Build history of the part. All positions in model axes, mm. A direction names the side the tool comes from. Coordinates: 2 decimals unless noted, no trailing zeros. Loops run counter-clockwise (first coordinate to the right, second up) from the corner with the lowest first, then second, coordinate; pieces in that order, holes last.
Item 1: 3-axis set-ups, long thin cutter, end or side, ignore diameter. For faces 1 (the face through (137, 40, -62)), 2 (the face through (-5, 65, 53)), 3 (the face through (19, 30, 1)), 4 (the face through (107, 40, 60)): which of +Z, -Z, +X, -X, +Y, -Y reach the whole face in a straight line?
Item 2: Cut at A-A (y = 47.5). List the corners of the cut face in (x, z), and give its area (3 significant figures).
Item 3: Cut at D-D (y = 17.5). List the corners of the cut face in (x, z), and give its area (3 significant figures).
Item 4: Cut at B-B (x = 45). List the corners of the cut face in (y, z), and give its area (3 significant figures).
Item 5: Drill centre lines: line 1 along X through (y, z) = (9, 13.5); line 2 along Y through (x, z) = (172, 9); line 3 along X through (y, z) = (-32.5, 14.5). Where is each one in solid material? Low to high.
Item 6: Cut at C-C (z = 33). List the corners of the cut face in (x, y), and give its area (3 significant figures).
Item 7: Mould opens along Y. For faces 5 (the face through (118, 35, 1)), 6 (the face through (167.5, 42.7, 62)), 7 (the face through (0, 15, 1)) say: released by +Y, released by -Y, zero draft, split by the parting line, or undercut.
Item 8: Flat gauge pins, fed straight in: pin 1 (1.5 mm diameter, centred on x = 83, z = 20.5, fed in from +Y); pin 2 (1.8 mm diameter, centred on x = 93.5, y = 41, fed in from -Z); pin 3 (5.5 mm diameter, centred on x = 183, y = 40, fed in from -Z); pin 4 (2.5 mm diameter, centred on x = 107.5, z = -63.5, fed in from -Y). Where does each tip first touch, or does it go through?
from build123d import *

# Parameters (mm, degrees)
EXTRUDE_1_DEPTH        = 65
SKETCH_5_W             = 5
SKETCH_5_H             = 5
CUT_EXTRUDE_1_DEPTH    = 3
SKETCH_7_W             = 5
SKETCH_7_H             = 23
EXTRUDE_2_DEPTH        = 40
FILLET_1_R             = 1
SKETCH_8_W             = 6
SKETCH_8_H             = 6
CUT_EXTRUDE_2_DEPTH    = 2
FILLET_1_OF_MIRROR_3_R = 1


with BuildPart() as part:
    # 草图1 → 凸台-拉伸1 (new body)
    with BuildSketch(Plane.XY):
        Polygon((190, 35), (190, 45), (-10, 45), (-10, 0), (0, 0), (0, 30), (39, 30), (39, -45), (49, -45), (49, 35), align=None)
    extrude_1 = extrude(amount=EXTRUDE_1_DEPTH)

    # 草图5 → 切除-拉伸1 (cut)
    with BuildSketch(Plane.XY.offset(65)):
        with Locations((167.5, 40)):
            Rectangle(SKETCH_5_W, SKETCH_5_H)
        with Locations((182.5, 40)):
            Rectangle(SKETCH_5_W, SKETCH_5_H)
        with Locations((152.5, 40)):
            Rectangle(SKETCH_5_W, SKETCH_5_H)
        with Locations((137.5, 40)):
            Rectangle(SKETCH_5_W, SKETCH_5_H)
        with Locations((122.5, 40)):
            Rectangle(SKETCH_5_W, SKETCH_5_H)
        with Locations((107.5, 40)):
            Rectangle(SKETCH_5_W, SKETCH_5_H)
        with Locations((92.5, 40)):
            Rectangle(SKETCH_5_W, SKETCH_5_H)
    cut_extrude_1 = extrude(amount=-CUT_EXTRUDE_1_DEPTH, mode=Mode.SUBTRACT)

    # 草图7 → 凸台-拉伸2 (add)
    with BuildSketch(Plane(origin=(0, 45, 0), x_dir=(1, 0, 0), z_dir=(0, 1, 0))):
        with Locations((-7.5, -53.5)):
            Rectangle(SKETCH_7_W, SKETCH_7_H)
    extrude_2 = extrude(amount=EXTRUDE_2_DEPTH)

    # 圆角1
    fillet_1_edges = [part.edges().sort_by_distance(p)[0] for p in [
        (-5, 65, 65),
        (-7.5, 85, 65),
        (-5, 0, 65),
        (0, 15, 65),
        (190, 45, 32.5),
        (190, 35, 32.5),
        (19.5, 30, 65),
        (39, -7.5, 65),
        (44, -45, 65),
        (49, -5, 65),
        (119.5, 35, 65),
        (190, 40, 65),
        (92.5, 45, 65),
        (-10, 42.5, 65),
    ]]
    fillet(fillet_1_edges, radius=FILLET_1_R)

    # 草图8 → 切除-拉伸2 (cut)
    with BuildSketch(Plane.XY.offset(62)):
        with Locations((182.5, 40)):
            Rectangle(SKETCH_8_W, SKETCH_8_H)
        with Locations((167.5, 40)):
            Rectangle(SKETCH_8_W, SKETCH_8_H)
        with Locations((152.5, 40)):
            Rectangle(SKETCH_8_W, SKETCH_8_H)
        with Locations((137.5, 40)):
            Rectangle(SKETCH_8_W, SKETCH_8_H)
        with Locations((122.5, 40)):
            Rectangle(SKETCH_8_W, SKETCH_8_H)
        with Locations((107.5, 40)):
            Rectangle(SKETCH_8_W, SKETCH_8_H)
        with Locations((92.5, 40)):
            Rectangle(SKETCH_8_W, SKETCH_8_H)
    extrude(amount=-CUT_EXTRUDE_2_DEPTH, mode=Mode.SUBTRACT)

    # 镜向3: 凸台-拉伸1, 切除-拉伸1, 凸台-拉伸2 across plane
    add(extrude_1.mirror(Plane.XY))
    add(cut_extrude_1.mirror(Plane.XY), mode=Mode.SUBTRACT)
    add(extrude_2.mirror(Plane.XY))

    # 圆角1 of 镜向3
    fillet_1_of_mirror_3_edges = [part.edges().sort_by_distance(p)[0] for p in [
        (-5, 65, -65),
        (-7.5, 85, -65),
        (-5, 0, -65),
        (0, 15, -65),
        (190, 45, -32.5),
        (190, 35, -32.5),
        (19.5, 30, -65),
        (39, -7.5, -65),
        (44, -45, -65),
        (49, -5, -65),
        (119.5, 35, -65),
        (190, 40, -65),
        (92.5, 45, -65),
        (-10, 42.5, -65),
    ]]
    fillet(fillet_1_of_mirror_3_edges, radius=FILLET_1_OF_MIRROR_3_R)


solid = part.part
Filled sheet:
1. face 1: -Z
1. face 2: +Z, -Z, +X, +Y
1. face 3: +Z, -Z, -Y
1. face 4: none
2. outline: (-10, -64) arc R1 ccw to (-9, -65) - (-6, -65) arc R1 ccw to (-5, -64) - (-5, -42) - (-10, -42) - close; (-10, 42) - (-5, 42) - (-5, 64) arc R1 ccw to (-6, 65) - (-9, 65) arc R1 ccw to (-10, 64) - close
2. area: 229 mm2
3. outline: (-10, -64) arc R1 ccw to (-9, -65) - (-1, -65) arc R1 ccw to (0, -64) - (0, 64) arc R1 ccw to (-1, 65) - (-9, 65) arc R1 ccw to (-10, 64) - close; (39, -64) arc R1 ccw to (40, -65) - (48, -65) arc R1 ccw to (49, -64) - (49, 64) arc R1 ccw to (48, 65) - (40, 65) arc R1 ccw to (39, 64) - close
3. area: 2,600 mm2
4. outline: (-45, -64) arc R1 ccw to (-44, -65) - (44, -65) arc R1 ccw to (45, -64) - (45, 64) arc R1 ccw to (44, 65) - (-44, 65) arc R1 ccw to (-45, 64) - close
4. area: 11,700 mm2
5. line 1: x = -10 to 0, 39 to 49
5. line 2: y = 35 to 45
5. line 3: x = 39 to 49
6. outline: (-10, 0) - (0, 0) - (0, 30) - (39, 30) - (39, -45) - (49, -45) - (49, 35) - (189, 35) arc R1 ccw to (190, 36) - (190, 44) arc R1 ccw to (189, 45) - (-10, 45) - close
6. area: 3,340 mm2
7. face 5: released by -Y
7. face 6: undercut
7. face 7: zero draft
8. pin 1: stops at y = 45
8. pin 2: stops at z = -62
8. pin 3: stops at z = -65
8. pin 4: stops at y = 35
